from build123d import *


with BuildPart() as f1:
    # F0 (on Front) → F1 (revolve)
    with BuildSketch(Plane.XZ):
        with BuildLine():
            Line((255.738805, 0), (0, 0))
            Line((0, 0), (0, -3.429))
            Line((0, -3.429), (256.737037, -3.429))
            Line((256.737037, -3.429), (270.505216, -14.083716))
            ThreePointArc((270.505216, -14.083716), (273.327727, -15.603563), (276.49007, -16.129))
            Line((276.49007, -16.129), (293.37, -16.129))
            Line((293.37, -16.129), (293.37, -12.7))
            Line((293.37, -12.7), (276.49007, -12.7))
            ThreePointArc((276.49007, -12.7), (274.4366, -12.358807), (272.603801, -11.371893))
            Line((272.603801, -11.371893), (259.625074, -1.328107))
            ThreePointArc((259.625074, -1.328107), (257.792275, -0.341193), (255.738805, 0))
        make_face()
    revolve(axis=Axis((0, 0, -1.7145), (0, 0, -1)))


solid = f1.part
CAD build for the part. Positions are in the model's coordinates, mm. A direction names the side the tool comes from. Round coordinates to 2 decimals unless told otherwise and drop trailing zeros. Order: outer loops, then holes, each group sorted by start corner. A loop starts at its lowest first (then second) coordinate and runs counter-clockwise, first axis right, second up. Notation, with made-up numbers: (20.25, 43) - (41.25, 43) arc R16 ccw to (41.25, 51) - close; hole circle Ø10 at (68.25, 49.25). An arc over 180 degrees is marked (long way). Return JSON: item names as keys, results as strings.
(1) Pull direction X, two halves, no side cores. Call faces 4 (the face through (197, -197, -16.129)), 5 (the face through (-38.191, -290.874, -14.39)), 6 (the face through (-55.842, 251.473, -4.096)): +X half, -X half, draft (parallel to the pull), parting line (faces both ways), or undercut.
Answer key:
{"face 4": "draft", "face 5": "parting line", "face 6": "undercut"}
(2) Pin check, flat tips, straight feed: pin 1 Ø4 at (x, y) = (-190.5, -182.5) entering from +Z; pin 2 Ø10 at (x, y) = (102, -232) entering from -Z; pin 3 Ø8 at (y, z) = (4.5, -5.5) entering from -X. Stop position of each tip, or through.
Answer key:
{"pin 1": "stops at z = -3.02", "pin 2": "stops at z = -4.74", "pin 3": "stops at x = -270.15"}
(3) Cut at A-A (y = 0). Give the cut face in (x, z).
Answer key:
{"outline": "(-293.37, -16.13) - (-276.49, -16.13) arc R9.78 ccw to (-270.51, -14.08) - (-256.74, -3.43) - (256.74, -3.43) - (270.51, -14.08) arc R9.78 ccw to (276.49, -16.13) - (293.37, -16.13) - (293.37, -12.7) - (276.49, -12.7) arc R6.35 cw to (272.6, -11.37) - (259.63, -1.33) arc R6.35 ccw to (255.74, 0) - (-255.74, 0) arc R6.35 ccw to (-259.63, -1.33) - (-272.6, -11.37) arc R6.35 cw to (-276.49, -12.7) - (-293.37, -12.7) - close"}
(4) Wall check: probe 1 along X at (y, z) = (-160, -9.75); probe 2 along Z at (x, y) = (135.5, -8); probe 3 along Y at (x, z) = (127, -3.5). Give the ranges that are in metal, low to high. Write a range as from..to.
Answer key:
{"probe 1": "x = -218.12..-211.13, 211.13..218.12", "probe 2": "z = -3.43..0", "probe 3": "y = -229.65..-223.23, 223.23..229.65"}
(5) Tool access for faces 1 (the face through (4, -4, -3.429)), 2 (the face through (-4, -4, 0)), 3 (the face through (-197, -197, -12.7)): list every direction of +Z, -Z, +X, -X, +Y, -Y with a clear straight run to the whole face (end or side of a thin tool).
Answer key:
{"face 1": "-Z", "face 2": "+Z, +X, -X, +Y, -Y", "face 3": "+Z"}
